Geometry check sheet. Reference: the model listing, model coordinates, mm. Face numbers are marked on the shaded views. Give positions to 0.01 mm unless a question says otherwise; leave off trailing zeros. Loops run counter-clockwise (first coordinate to the right, second up) from the corner with the lowest first, then second, coordinate; pieces in that order, holes last. Notation, with made-up numbers: (4.5, -9) -> (24.5, -9) arc R30 ccw to (24.5, 17) -> close; hole circle Ø8 at (88, 25.25). An arc over 180 degrees is marked (long way). Write item = value, one per line. Start each with the question number.
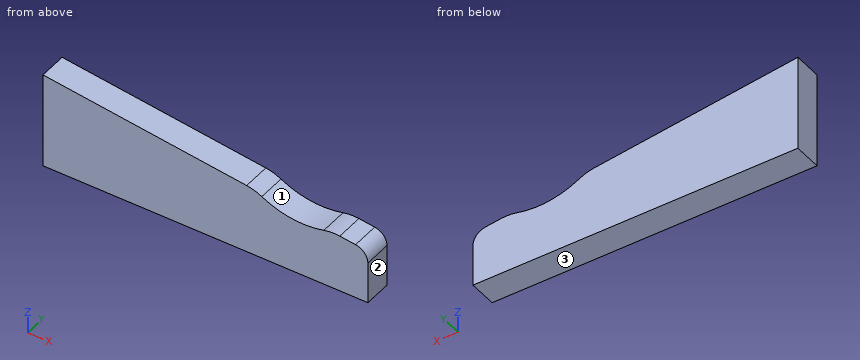
Solid Edge part; units mm, degrees
sketch "Sketch1" plane through (0, 0, 0) normal (0, -1, 0) x (1, 0, 0)
  line L0 (0, 0) -> (115, 0)
  line L1 (115, 0) -> (115, -34)
  line L2 (115, -34) -> (0, -34)
  line L3 (0, -34) -> (0, 0)
extrude "Protrusion1" add sketch "Sketch1" against normal blind 10
sketch "Sketch2" plane through (57.5, 0, -17) normal (0, -1, 0) x (1, 0, 0)
  line L0 (57.5, 2.2) -> (-57.5, 17)
  line L1 (-57.5, 17) -> (57.5, 17)
  line L2 (57.5, 17) -> (57.5, 2.2)
extrude "ExtrudedCutout_1" cut sketch "Sketch2" against normal blind 10
sketch "Sketch3" plane through (57.5, 0, -17) normal (0, -1, 0) x (1, 0, 0)
  circle A0 centre (34.5, 32.2) radius 30
extrude "ExtrudedCutout_2" cut sketch "Sketch3" against normal blind 10
fillet "Round_1" radius 15 2 edges at (75.2424, 5, -9.6834) (101.9112, 5, -13.1155)
fillet "Round_3" radius 5 1 edges at (115, 5, -14.8)
1) Section check B-B (x = 65). Enter the section's corners in (y, z), plus the area to 3 significant figures.
2) Depth check by flat-ended pin: pin 1 Ø1.5 at (x, y) = (74.5, 6) entering from +Z. Enter the tip coordinate at first touch or a pass-through.
3) Section check C-C (z = -12). Enter the section's corners in (x, y), plus the area to 3 significant figures.
4) Thickness scan on line 1 (Z direction, x = 24, y = 4.75); line 2 (Z direction, x = 79, y = 2.25); line 3 (X direction, y = 5.75, z = -16). Record the ranges inside material, lowest first.
5) Section check A-A (y = 8). Enter the section's corners in (x, z).
6) Draft check along X on the marked faces 1, 2 and 3. Enter one of: released by +X, released by -X, zero draft, split by the parting line, or undercut.
Check result:
q1.outline = (0, -34) -> (10, -34) -> (10, -8.37) -> (0, -8.37) -> close
q1.area = 256 mm2
q2.pin_1 = -9.59
q3.outline = (0, 0) -> (79.34, 0) -> (79.34, 10) -> (0, 10) -> close
q3.area = 793 mm2
q4.line_1 = -34 to -3.09
q4.line_2 = -34 to -11.84
q4.line_3 = 0 to 113.84
q5.outline = (0, -34) -> (115, -34) -> (115, -19.2) arc R5 ccw to (110.64, -14.24) -> (105.06, -13.52) arc R15 ccw to (99.43, -13.87) arc R30 cw to (77.45, -11.04) arc R15 ccw to (72.09, -9.28) -> (0, 0) -> close
q6.face_1 = undercut
q6.face_2 = released by +X
q6.face_3 = zero draft
